Can you work these out from the drawing? Everything is in mm from the part's minimum corner. Give positions to 0.01 mm unless a question says otherwise; leave off trailing zeros. Loops run counter-clockwise (first coordinate to the right, second up) from the corner with the lowest first, then second, coordinate; pieces in that order, holes last.
Q1. Will this pin go through, and if not, where does the flat tip stop? P1, Ø3, axis at x = 129, y = 105, coming from the +Z side.
Q2. If we section it at B-B (y = 105): Please give me the cut outline in (x, z), plus the area to 3 significant figures.
Q3. I need wall thicknesses on line 1 (Y direction, x = 15, z = 1.65); line 2 (X direction, y = 119, z = 1.55). Which ranges of each line are inside material? Lowest first, please.
Q4. If we section it at A-A (x = 140): Please give me the cut outline in (y, z), plus the area to 3 significant figures.
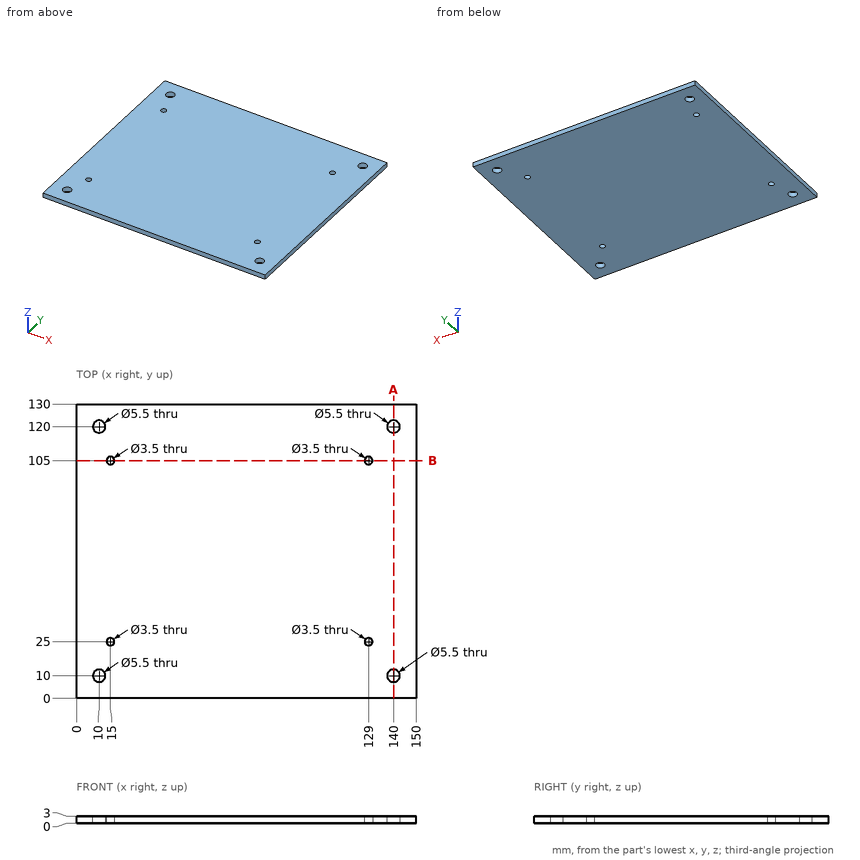
Check sheet entries:
1. P1: passes through
2. outline: (0, 0) - (13.25, 0) - (13.25, 3) - (0, 3) - close; (16.75, 0) - (127.25, 0) - (127.25, 3) - (16.75, 3) - close; (130.75, 0) - (150, 0) - (150, 3) - (130.75, 3) - close
2. area: 429 mm2
3. line 1: y = 0 to 23.25, 26.75 to 103.25, 106.75 to 130
3. line 2: x = 0 to 7.44, 12.56 to 137.44, 142.56 to 150
4. outline: (0, 0) - (7.25, 0) - (7.25, 3) - (0, 3) - close; (12.75, 0) - (117.25, 0) - (117.25, 3) - (12.75, 3) - close; (122.75, 0) - (130, 0) - (130, 3) - (122.75, 3) - close
4. area: 357 mm2
